The listing builds one solid part. Answer for the finished solid, in the listing's coordinates (mm). A direction names the side the tool comes from. Give positions to 0.01 mm unless a question says otherwise; leave off trailing zeros. Write each loop counter-clockwise with the first axis right and the second up, starting at its lowest first coordinate (ties: lowest second). Pieces come first, ordered by that corner, then holes. Notation, with made-up numbers: (-38.75, 70.5) -> (10.25, 70.5) arc R20 ccw to (10.25, 98.5) -> close; hole circle Ø3 at (14, 65). An arc over 180 degrees is marked (long way). Put each result on its own line as item: value. Start each with the question number.
1) For faces 4 (the flat face through (5, 12, 0)), 5 (the flat face through (30, 12, 18)), determine the directions among +Z, -Z, +X, -X, +Y, -Y from which every point of the face is accessible in a straight line to the end or side of a thin tool.
2) A cutting plane is placed at B-B (y = 11). Write down the section's boundary in (x, z), then the cut area to 3 significant figures.
3) Flat-ended cylindrical pins translate along their axes: pin 1 Ø12.5 at (y, z) = (10, 5.5) entering from +X; pin 2 Ø5 at (x, y) = (46.5, 12.5) entering from -Z; pin 3 Ø3 at (y, z) = (5.5, -12.5) entering from +X; pin 4 Ø10 at (y, z) = (7, -12.5) entering from +X. Find the tip coordinate at first contact, or state that the pin passes through.
4) For a pull along X with two mould halves and no side action, classify faces 1 (the cylindrical face through (42.504, 12.676, 15.535)), 2 (the flat face through (31, 12, -18)), 3 (the cylindrical face through (55.436, 3.759, 15.465)) as released by +X, released by -X, zero draft, split by the parting line, or undercut.
5) Find the intervals of material crossed by line 1 along Z through (x, y) = (14, 2.5); line 2 along Y through (x, z) = (46.5, -15.55); line 3 along X through (y, z) = (8, -8.5), in increasing order. Write a range as from..to.
6) A cutting plane is placed at D-D (z = -11). Write down the section's boundary in (x, y).
7) A cutting plane is placed at A-A (x = 12.5). Write down the section's boundary in (y, z).
8) A cutting plane is placed at C-C (y = 6). Write down the section's boundary in (x, z), then the cut area to 3 significant figures.
from build123d import *

# Parameters (mm, degrees)
EXTRUDE_1_DEPTH     = 25
FILLET_1_R          = 12.5
SKETCH_2_R          = 4
CUT_EXTRUDE_1_DEPTH = 74.4982993


with BuildPart() as part:
    # Эскиз1 → Бобышка-Вытянуть1 (new body)
    with BuildSketch(Plane(origin=(0, 0, 0), x_dir=(1, 0, 0), z_dir=(0, 1, 0))):
        with BuildLine():
            Line((0, 16), (0, -16))
            ThreePointArc((0, -16), (0.585786438, -17.414213562), (2, -18))
            Line((2, -18), (59, -18))
            Line((59, -18), (59, -13))
            Line((59, -13), (5, -13))
            Line((5, -13), (5, 13))
            Line((5, 13), (59, 13))
            Line((59, 13), (59, 18))
            Line((59, 18), (2, 18))
            ThreePointArc((2, 18), (0.585786438, 17.414213562), (0, 16))
        make_face()
    extrude(amount=EXTRUDE_1_DEPTH)

    # Скругление1
    fillet_1_edges = [part.edges().sort_by_distance(p)[0] for p in [
        (59, 25, -15.5),
        (59, 0, -15.5),
        (59, 0, 15.5),
        (59, 25, 15.5),
    ]]
    fillet(fillet_1_edges, radius=FILLET_1_R - 0.0001)  # a hair under: the kernel refuses the full size

    # Эскиз2 → Вырез-Вытянуть1 (cut, through all)
    with BuildSketch(Plane.XY.offset(18)):
        with Locations((46.5, 12.5)):
            Circle(SKETCH_2_R)
    extrude(amount=-CUT_EXTRUDE_1_DEPTH, mode=Mode.SUBTRACT)


solid = part.part
Reply:
1. face 4: +X, +Y, -Y
1. face 5: +Z, +X, -X, +Y, -Y
2. outline: (0, -16) arc R2 ccw to (2, -18) -> (42.79, -18) -> (42.79, -13) -> (5, -13) -> (5, 13) -> (42.79, 13) -> (42.79, 18) -> (2, 18) arc R2 ccw to (0, 16) -> close; (50.21, -18) -> (58.91, -18) -> (58.91, -13) -> (50.21, -13) -> close; (50.21, 13) -> (58.91, 13) -> (58.91, 18) -> (50.21, 18) -> close
2. area: 643 mm2
3. pin 1: stops at x = 5
3. pin 2: passes through
3. pin 3: stops at x = 57.68
3. pin 4: stops at x = 58.99
4. face 1: undercut
4. face 2: zero draft
4. face 3: released by +X
5. line 1: z = -18..-13, 13..18
5. line 2: y = 0..8.5, 16.5..25
5. line 3: x = 0..5
6. outline: (0, 0) -> (5, 0) -> (5, 25) -> (0, 25) -> close
7. outline: (0, -18) -> (25, -18) -> (25, -13) -> (0, -13) -> close; (0, 13) -> (25, 13) -> (25, 18) -> (0, 18) -> close
8. outline: (0, -16) arc R2 ccw to (2, -18) -> (57.18, -18) -> (57.18, -13) -> (5, -13) -> (5, 13) -> (57.18, 13) -> (57.18, 18) -> (2, 18) arc R2 ccw to (0, 16) -> close
8. area: 700 mm2
